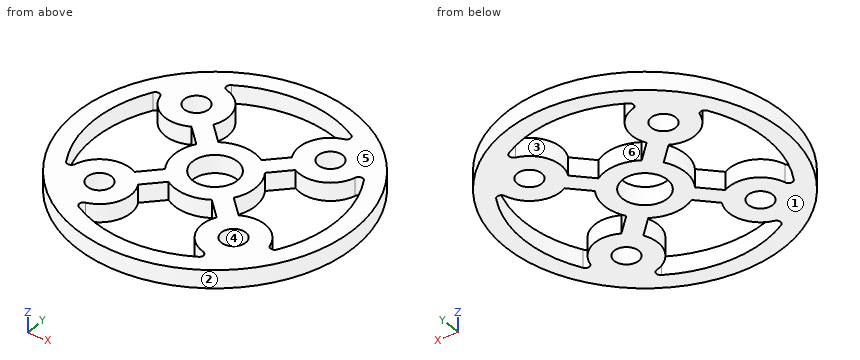
```python
from build123d import *

# Parameters (mm, degrees)
F0_R            = 24.51608
F0_R_2          = 2.15265
F0_R_3          = 3.96875
F1_DEPTH        = 3.175
F3_DEPTH        = 3.175
F3_COPIES_COUNT = 4
F4_R            = 0.762


# Not quite as in the source:
# - a pattern or mirror of a feature is missing from the dataset's text; its kind, count and spacing are read off the source's solid


with BuildPart() as f1:
    # F0 (on Top) → F1 (new body)
    with BuildSketch(Plane.XY):
        Circle(F0_R)
        with Locations((-11.7865906, -11.7865906)):
            Circle(F0_R_2, mode=Mode.SUBTRACT)
        with Locations((11.7865906, -11.7865906)):
            Circle(F0_R_2, mode=Mode.SUBTRACT)
        with Locations((-11.7865906, 11.7865906)):
            Circle(F0_R_2, mode=Mode.SUBTRACT)
        Circle(F0_R_3, mode=Mode.SUBTRACT)
        with Locations((11.7865906, 11.7865906)):
            Circle(F0_R_2, mode=Mode.SUBTRACT)
    extrude(amount=F1_DEPTH)

    # F2 (on face) → F3 (cut, through all)
    with BuildSketch(Plane.XY.offset(3.175)):
        with BuildLine():
            ThreePointArc((-12.5005198818, 17.2967828873), (-7.207099086, 14.9330444032), (-6.8989717457, 9.144035776))
            Line((-6.8989717457, 9.144035776), (-3.8025572131, 6.0476212434))
            ThreePointArc((-3.8025572131, 6.0476212434), (0, 7.14375), (3.8025572131, 6.0476212434))
            Line((3.8025572131, 6.0476212434), (6.8989717457, 9.144035776))
            ThreePointArc((6.8989717457, 9.144035776), (7.207099086, 14.9330444032), (12.5005198818, 17.2967828873))
            ThreePointArc((12.5005198818, 17.2967828873), (0, 21.34108), (-12.5005198818, 17.2967828873))
        make_face()
    f3 = extrude(amount=-F3_DEPTH, mode=Mode.SUBTRACT)

    # F3_copies: F3 ×4 about axis
    f3_copies_axis = Axis((0, 0, 0), (0, 0, 1))
    for i in range(1, F3_COPIES_COUNT):
        add(f3.rotate(f3_copies_axis, i * 360 / F3_COPIES_COUNT), mode=Mode.SUBTRACT)

    # F4
    f4_edges = [f1.edges().sort_by_distance(p)[0] for p in [
        (-12.50052, 17.296783, 1.5875),
        (12.50052, 17.296783, 1.5875),
        (12.50052, -17.296783, 1.5875),
        (-12.50052, -17.296783, 1.5875),
        (17.296783, 12.50052, 1.5875),
        (17.296783, -12.50052, 1.5875),
        (-17.296783, -12.50052, 1.5875),
        (-17.296783, 12.50052, 1.5875),
    ]]
    fillet(f4_edges, radius=F4_R)


solid = f1.part
```
CAD build for the part. Positions are in the model's coordinates, mm. Face numbers are marked on the shaded views. A direction names the side the tool comes from. Round coordinates to 2 decimals unless told otherwise and drop trailing zeros. Loops run counter-clockwise (first coordinate to the right, second up) from the corner with the lowest first, then second, coordinate; pieces in that order, holes last. Notation, with made-up numbers: (-6, 37.25) - (52, 37.25) arc R24 ccw to (52, 52.25) - close; hole circle Ø1 at (41, -1). An arc over 180 degrees is marked (long way). Return JSON: item names as keys, results as strings. Group by question number.
Q1. Band-saw the part on C-C on y = 15. Give the cut face in (x, z) (3 decimals).
Q2. Two-plate mould, pull along X, no slides. Class the marked faces 1, 2, 3 and 4: +X half, -X half, draft (parallel to the pull), parting line (faces both ways), or undercut.
Q3. Drill centre lines: line 1 along X through (y, z) = (3, 2.5); line 2 along X through (y, z) = (-10.5, 2.8); line 3 along X through (y, z) = (10, 2.6). Where is each one in solid material? Low to high. Write a range as [from, to].
Q4. Band-saw the part on A-A on x = 0. Give the cut face in (y, z) (3 decimals), plus the area to 3 significant figures.
Q5. Band-saw the part on D-D on z = 0.8. Give the number of separate pieces and of enclosed holes in the cut face, plus the area to 3 significant figures.
Q6. Tool access for the marked faces 5 and 6: list every direction of +Z, -Z, +X, -X, +Y, -Y with a clear straight run to the whole face (end or side of a thin tool).
Q7. Flat gauge pins, fed straight in: pin 1 Ø1 at (x, y) = (-6.5, -16.5) entering from +Z; pin 2 Ø1 at (x, z) = (15, 2.5) entering from +Y; pin 3 Ø1.5 at (y, z) = (-11.5, 1) entering from -X. Where does each tip first touch, or does it go through?
Solutions:
{
 "1": {"outline": "(-19.392, 0) - (-7.254, 0) - (-7.254, 3.175) - (-19.392, 3.175) - close; (7.254, 0) - (19.392, 0) - (19.392, 3.175) - (7.254, 3.175) - close"},
 "2": {"face 1": "draft", "face 2": "parting line", "face 3": "undercut", "face 4": "undercut"},
 "3": {"line 1": "x = [-24.33, -21.13], [-6.48, -2.6], [2.6, 6.48], [21.13, 24.33]", "line 2": "x = [-22.15, -18.58], [-17.21, -13.51], [-10.06, -6.38], [6.38, 10.06], [13.51, 17.21], [18.58, 22.15]", "line 3": "x = [-22.38, -18.85], [-17.05, -12.99], [-10.59, -6.53], [6.53, 10.59], [12.99, 17.05], [18.85, 22.38]"},
 "4": {"outline": "(-24.516, 0) - (-21.341, 0) - (-21.341, 3.175) - (-24.516, 3.175) - close; (-7.144, 0) - (-3.969, 0) - (-3.969, 3.175) - (-7.144, 3.175) - close; (3.969, 0) - (7.144, 0) - (7.144, 3.175) - (3.969, 3.175) - close; (21.341, 0) - (24.516, 0) - (24.516, 3.175) - (21.341, 3.175) - close", "area": "40.3 mm^2"},
 "5": {"separate pieces": "1", "enclosed holes": "9", "area": "941 mm^2"},
 "6": {"face 5": "+Z, +X, -X, +Y, -Y", "face 6": "+Z, -Z"},
 "7": {"pin 1": "passes through", "pin 2": "stops at y = 19.77", "pin 3": "stops at x = -22.03"}
}
